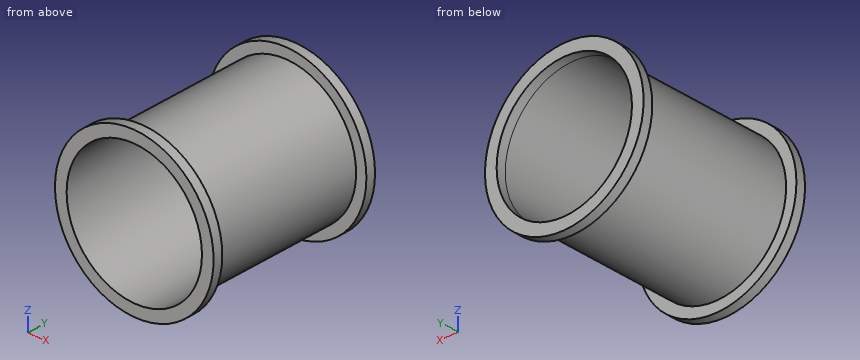
Autodesk Inventor part; units mm, degrees
ref_plane "YZ Plane" through (0, 0, 0) normal (1, 0, 0) x (0, 1, 0)
ref_plane "XZ Plane" through (0, 0, 0) normal (0, 1, 0) x (-1, 0, 0)
ref_plane "XY Plane" through (0, 0, 0) normal (0, 0, 1) x (1, 0, 0)
sketch "Sketch1" plane through (0, 0, 0) normal (0, 1, 0) x (-1, 0, 0)
  circle A0 centre (0, 0) radius 184.15
  circle A1 centre (0, 0) radius 215.9
  dimension "d0" = 368.3
  dimension "d1" = 431.8
extrude "Extrusion1" add sketch "Sketch1" along normal blind 25.4
sketch "Sketch2" plane through (0, 25.4, 0) normal (0, 1, 0) x (1, 0, 0)
  circle A0 centre (0, 0) radius 184.15
  circle A1 centre (0, 0) radius 187.96
  dimension "d4" = 368.3
  dimension "d5" = 375.92
extrude "Extrusion2" add sketch "Sketch2" along normal blind 423.8625
sketch "Sketch3" plane through (0, 449.2625, 0) normal (0, 1, 0) x (1, 0, 0)
  circle A0 centre (0, 0) radius 184.15
  circle A1 centre (0, 0) radius 215.9
  dimension "d8" = 368.3
  dimension "d9" = 431.8
extrude "Extrusion3" add sketch "Sketch3" along normal blind 25.4
properties part number "Radiation Sheild 55K" material "Aluminum 6061"
For this review, take the finished solid that the model builds, in its own axes (mm). Coordinates: 2 decimals unless noted, no trailing zeros. Order: outer loops, then holes, each group sorted by start corner. A loop starts at its lowest first (then second) coordinate and runs counter-clockwise, first axis right, second up. Notation, with made-up numbers: (42, 15) -> (70, 15) arc R25 ccw to (70, 51) -> close; hole circle Ø9 at (31.25, 69.25). An arc over 180 degrees is marked (long way). Answer as CSV lines item,"result".
Q1. Wall thickness on line 1 along Z through (x, y) = (0, 468); line 2 along Z through (x, y) = (3.5, 448): over which ranges is each line inside the solid? List them lowest first. Write a range as [from, to].
Model answer:
line 1,"z = [-215.9, -184.15], [184.15, 215.9]"
line 2,"z = [-187.93, -184.12], [184.12, 187.93]"
Q2. We need section C-C (y = 349). State the section outline as (x, z) points, plus the area to 3 significant figures.
Model answer:
outline,"circle Ø375.92 at (0, 0); hole circle Ø368.3 at (0, 0)"
area,"4,450 mm2"
Q3. Clearance check with flat-ended pins moving along their axes: pin 1 Ø5 at (y, z) = (352.5, 38) entering from +X; pin 2 Ø6 at (x, y) = (-6.5, 322) entering from -Z; pin 3 Ø1 at (x, y) = (-132, 236) entering from +Z. State where each tip first meets the part, or that it passes through.
Model answer:
pin 1,"stops at x = 184.58"
pin 2,"stops at z = -187.93"
pin 3,"stops at z = 134.3"
Q4. We need section A-A (z = -54). State the section outline as (x, y) points.
Model answer:
outline,"(-209.04, 0) -> (-176.05, 0) -> (-176.05, 474.66) -> (-209.04, 474.66) -> (-209.04, 449.26) -> (-180.04, 449.26) -> (-180.04, 25.4) -> (-209.04, 25.4) -> close; (176.05, 0) -> (209.04, 0) -> (209.04, 25.4) -> (180.04, 25.4) -> (180.04, 449.26) -> (209.04, 449.26) -> (209.04, 474.66) -> (176.05, 474.66) -> close"
